Autodesk Inventor part; units mm, degrees
ref_plane "YZ Plane" through (0, 0, 0) normal (1, 0, 0) x (0, 1, 0)
ref_plane "XZ Plane" through (0, 0, 0) normal (0, 1, 0) x (-1, 0, 0)
ref_plane "XY Plane" through (0, 0, 0) normal (0, 0, 1) x (1, 0, 0)
sketch "スケッチ1" plane through (0, 0, 0) normal (0, 0, 1) x (1, 0, 0)
  circle A0 centre (0, 0) radius 12.8
  circle A1 centre (0, 11) radius 1.35
  circle A2 centre (7.7782, 7.7782) radius 1.35
  circle A3 centre (11, 0) radius 1.35
  circle A4 centre (7.7782, -7.7782) radius 1.35
  circle A5 centre (0, -11) radius 1.35
  circle A6 centre (-7.7782, -7.7782) radius 1.35
  circle A7 centre (-11, 0) radius 1.35
  circle A8 centre (-7.7782, 7.7782) radius 1.35
  circle A9 centre (0, 0) radius 5
  circle A10 centre (0, 8) radius 1
  circle A11 centre (-8, 0) radius 1
  circle A12 centre (8, 0) radius 1
  circle A13 centre (0, -8) radius 1
  circle A14 centre (0, 0) radius 6
  circle A15 centre (0, 0) radius 13.5
  circle A16 centre (0, 11) radius 1.75
  circle A17 centre (-11, 0) radius 1.75
  circle A18 centre (0, -11) radius 1.75
  circle A19 centre (11, 0) radius 1.75
  point P0 (0, 0)
  dimension "d0" = 12
  dimension "d1" = 27
  dimension "d2" = 3.5
  dimension "d3" = 3.5
  dimension "d4" = 3.5
  dimension "d5" = 3.5
extrude "押し出し1" add sketch "スケッチ1" along normal blind 3.2 contours A0 | A2 | A4 | A6 | A8 | A10 | A11 | A12 | A13 | A15
The model under review builds one solid part; all positions refer to its coordinate system, in mm. Round coordinates to 2 decimals unless told otherwise and drop trailing zeros. Order: outer loops, then holes, each group sorted by start corner. A loop starts at its lowest first (then second) coordinate and runs counter-clockwise, first axis right, second up. Notation, with made-up numbers: (48.25, 74.25) -> (67.25, 74.25) arc R22 cw to (67.25, 92.25) -> close; hole circle Ø2 at (-33, 29.25). An arc over 180 degrees is marked (long way). One line per item, written item: value. Start each with the question number.
Q1. Take a section at C-C (x = -11). Write out the cut boundary in (y, z), and give its area (3 significant figures).
Q2. Mouldability with a two-part tool opening along Y and no side actions: class faces 1 (the face through (-9.331, -0.526, 1.578)), 2 (the face through (6, -3, 3.2)), 3 (the face through (-2.93, 13.18, 1.58)) as released by +Y, released by -Y, zero draft, split by the parting line, or undercut.
Q3. Take a section at B-B (y = -4.25). Write out the cut boundary in (x, z).
Q4. Wall thickness on line 1 (Y direction, x = 0, z = 1.6); line 2 (X direction, y = 1.5, z = 2.8); line 3 (X direction, y = -1.25, z = 2.45): over which ranges is each line inside the solid? List them lowest first.
Q5. Clearance check with flat-ended pins moving along their axes: pin 1 Ø12 at (x, y) = (-10.5, 7) entering from -Z; pin 2 Ø1.5 at (y, z) = (-7, 2.5) entering from -X; pin 3 Ø1 at (x, z) = (-6, 2) entering from +Y; pin 4 Ø3 at (x, y) = (-11, 0) entering from -Z. State where each tip first meets the part, or that it passes through.
Q6. Take a section at A-A (x = 0). Write out the cut boundary in (y, z).
Q7. Take a section at D-D (z = 2.7). Write out the cut boundary in (x, y), and give its area (3 significant figures).
Reported:
1. outline: (-7.83, 0) -> (-1.75, 0) -> (-1.75, 3.2) -> (-7.83, 3.2) -> close; (1.75, 0) -> (7.83, 0) -> (7.83, 3.2) -> (1.75, 3.2) -> close
1. area: 38.9 mm2
2. face 1: undercut
2. face 2: zero draft
2. face 3: split by the parting line
3. outline: (-12.81, 0) -> (-4.24, 0) -> (-4.24, 3.2) -> (-12.81, 3.2) -> close; (4.24, 0) -> (12.81, 0) -> (12.81, 3.2) -> (4.24, 3.2) -> close
4. line 1: y = -13.5 to -12.75, -9.25 to -6, 6 to 9.25, 12.75 to 13.5
4. line 2: x = -13.42 to -11.9, -10.1 to -5.81, 5.81 to 10.1, 11.9 to 13.42
4. line 3: x = -13.44 to -12.22, -9.78 to -5.87, 5.87 to 9.78, 12.22 to 13.44
5. pin 1: stops at z = 0
5. pin 2: stops at x = -11.97
5. pin 3: stops at y = 12.33
5. pin 4: passes through
6. outline: (-13.5, 0) -> (-12.75, 0) -> (-12.75, 3.2) -> (-13.5, 3.2) -> close; (-9.25, 0) -> (-6, 0) -> (-6, 3.2) -> (-9.25, 3.2) -> close; (6, 0) -> (9.25, 0) -> (9.25, 3.2) -> (6, 3.2) -> close; (12.75, 0) -> (13.5, 0) -> (13.5, 3.2) -> (12.75, 3.2) -> close
7. outline: circle Ø27 at (0, 0); hole circle Ø3.5 at (-11, 0); hole circle Ø12 at (0, 0); hole circle Ø3.5 at (0, -11); hole circle Ø3.5 at (0, 11); hole circle Ø3.5 at (11, 0)
7. area: 421 mm2
